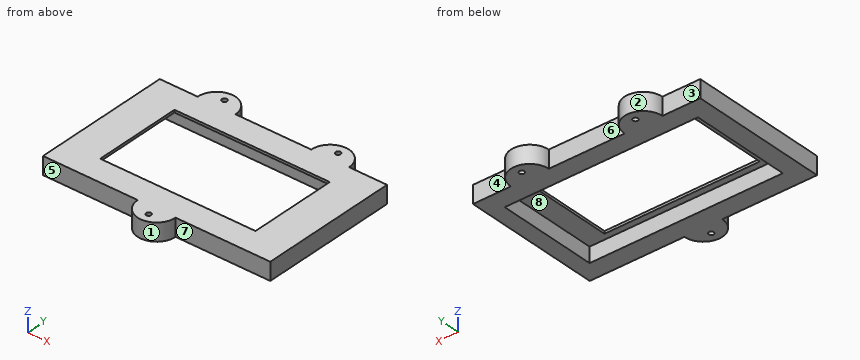
from build123d import *

# Parameters (mm, degrees)
F0_R      = 2
F1_DEPTH  = 25
F3_DEPTH  = 276
F4_R      = 2
F5_DEPTH  = 84.8
F6_R      = 2.5
F7_DEPTH  = 5
F9_DEPTH  = 14
F11_W     = 123
F11_H     = 70
F12_DEPTH = 25
F13_W     = 153
F13_H     = 80
F14_DEPTH = 12
F15_R     = 2
F16_DEPTH = 25


with BuildPart() as f1:
    # F0 (on Top) → F1 (new body)
    with BuildSketch(Plane.XY):
        with BuildLine():
            Line((-51.434658, 66.572686), (-81.434658, 66.572686))
            Line((-81.434658, 66.572686), (-81.434658, -43.427314))
            Line((-81.434658, -43.427314), (-6.434658, -43.427314))
            ThreePointArc((-6.434658, -43.427314), (8.565342, -58.427314), (23.565342, -43.427314))
            Line((23.565342, -43.427314), (98.565342, -43.427314))
            Line((98.565342, -43.427314), (98.565342, 66.572686))
            Line((98.565342, 66.572686), (68.565342, 66.572686))
            ThreePointArc((68.565342, 66.572686), (53.565342, 81.572686), (38.565342, 66.572686))
            Line((38.565342, 66.572686), (-21.434658, 66.572686))
            ThreePointArc((-21.434658, 66.572686), (-36.434658, 81.572686), (-51.434658, 66.572686))
        make_face()
        with Locations((8.565342, -50.927314)):
            Circle(F0_R, mode=Mode.SUBTRACT)
        with Locations((-36.434658, 74.072686)):
            Circle(F0_R, mode=Mode.SUBTRACT)
        with Locations((53.565342, 74.072686)):
            Circle(F0_R, mode=Mode.SUBTRACT)
    extrude(amount=F1_DEPTH)

    # F2 (on face) → F3 (cut)
    with BuildSketch(Plane.YZ.offset(98.565342)):
        with BuildLine():
            Line((43.145373, 0), (22.822686, 0))
            ThreePointArc((22.822686, 0), (11.572686, 11.25), (0.322686, 0))
            Line((0.322686, 0), (-20, 0))
            ThreePointArc((-20, 0), (-41.231841, 11.150842), (-64.902842, 15))
            Line((-64.902842, 15), (-64.902842, -16.413443))
            Line((-64.902842, -16.413443), (88.048215, -16.413443))
            Line((88.048215, -16.413443), (88.048215, 15))
            ThreePointArc((88.048215, 15), (64.377213, 11.150842), (43.145373, 0))
        make_face()
    extrude(amount=-F3_DEPTH, mode=Mode.SUBTRACT)

    # F4 (on face) → F5 (cut)
    with BuildSketch(Plane.XY.offset(25)):
        with Locations((-56.434658, 32.872686)):
            Circle(F4_R)
        with Locations((73.565342, 32.872686)):
            Circle(F4_R)
        with Locations((-56.434658, -9.727314)):
            Circle(F4_R)
        with Locations((73.565342, -9.727314)):
            Circle(F4_R)
    extrude(amount=-F5_DEPTH, mode=Mode.SUBTRACT)

    # F6 (on face) → F7 (cut)
    with BuildSketch(Plane.XY.offset(25)):
        with Locations((-56.434658, 32.872686)):
            Circle(F6_R)
        with Locations((73.565342, 32.872686)):
            Circle(F6_R)
        with Locations((73.565342, -9.727314)):
            Circle(F6_R)
        with Locations((-56.434658, -9.727314)):
            Circle(F6_R)
    extrude(amount=-F7_DEPTH, mode=Mode.SUBTRACT)


with BuildPart() as f9:
    # F8 (on face) → F9 (new body)
    with BuildSketch(Plane.XY.offset(25)):
        with BuildLine():
            Line((-81.434658, -43.427314), (-6.434658, -43.427314))
            ThreePointArc((-6.434658, -43.427314), (8.565342, -58.427314), (23.565342, -43.427314))
            Line((23.565342, -43.427314), (98.565342, -43.427314))
            Line((98.565342, -43.427314), (98.565342, 66.572686))
            Line((98.565342, 66.572686), (68.565342, 66.572686))
            ThreePointArc((68.565342, 66.572686), (53.565342, 81.572686), (38.565342, 66.572686))
            Line((38.565342, 66.572686), (-21.434658, 66.572686))
            ThreePointArc((-21.434658, 66.572686), (-36.434658, 81.572686), (-51.434658, 66.572686))
            Line((-51.434658, 66.572686), (-81.434658, 66.572686))
            Line((-81.434658, 66.572686), (-81.434658, -43.427314))
        make_face()
    extrude(amount=F9_DEPTH)

    # F11 (on face) → F12 (cut)
    with BuildSketch(Plane.XY.offset(39)):
        with Locations((8.565342, 11.572686)):
            Rectangle(F11_W, F11_H)
    extrude(amount=-F12_DEPTH, mode=Mode.SUBTRACT)

    # F13 (on face) → F14 (cut)
    with BuildSketch(Plane(origin=(0, 0, 25), x_dir=(1, 0, 0), z_dir=(0, 0, -1))):
        with Locations((9.565342, -11.572686)):
            Rectangle(F13_W, F13_H)
    extrude(amount=-F14_DEPTH, mode=Mode.SUBTRACT)

    # F15 (on face) → F16 (cut)
    with BuildSketch(Plane.XY.offset(39)):
        with Locations((53.565342, 74.072686)):
            Circle(F15_R)
        with Locations((-36.434658, 74.072686)):
            Circle(F15_R)
        with Locations((8.565342, -50.927314)):
            Circle(F15_R)
    extrude(amount=-F16_DEPTH, mode=Mode.SUBTRACT)


solid = f9.part
The model under review builds one solid part; all positions refer to its coordinate system, in mm. Face numbers are marked on the shaded views. A direction names the side the tool comes from. Give positions to 0.01 mm unless a question says otherwise; leave off trailing zeros. Order: outer loops, then holes, each group sorted by start corner. A loop starts at its lowest first (then second) coordinate and runs counter-clockwise, first axis right, second up. Notation, with made-up numbers: M -11.75,63.25 L 6.25,63.25 A6 cw 6.25,68.25 Z; hole C 35,50.25 d9. An arc over 180 degrees is marked long. Answer in a Markdown table with one row per item. Add a question column.
1. Add section A-A on y = 22. State the section outline as (x, z) points, plus the area to 3 significant figures.
2. Add section D-D on x = -60. State the section outline as (y, z) points, plus the area to 3 significant figures.
3. To check wall thickness, follow line 1 along X through (y, z) = (9, 30.5); line 2 along Y through (x, z) = (-8, 30.25); line 3 along Y through (x, z) = (52, 30.25). State the ranges of each line that lie inside material, in increasing order.
4. Mouldability with a two-part tool opening along X and no side actions: class the marked faces 1, 2 and 3 as released by +X, released by -X, zero draft, split by the parting line, or undercut.
5. Machinability: for the marked faces 4, 5, 6, 7 and 8, which of the approach directions +Z, -Z, +X, -X, +Y, -Y give a long, thin tool a straight path to every point of the face, cutting with its end or side? Answer none if there is none.
6. Add section C-C on z = 32. State the section outline as (x, y) points.
7. Add section B-B on x = 63. State the section outline as (y, z) points, plus the area to 3 significant figures.
8. For pin 1 Ø7 at (x, z) = (-35.5, 29) entering from -Y; pin 2 Ø0.6 at (x, z) = (-6.5, 38) entering from +Y; pin 3 Ø1 at (x, z) = (17, 36) entering from -Y; pin 4 Ø2.5 at (x, y) = (8.57, -50.93) entering from -Z, all flat-tipped, find the tip position at first contact; note any pin that passes through.
The answers:
| question | item | result |
|---|---|---|
| 1 | outline | M -81.43,25 L -66.93,25 L -66.93,37 L -52.93,37 L -52.93,39 L -81.43,39 Z; M 70.07,37 L 86.07,37 L 86.07,25 L 98.57,25 L 98.57,39 L 70.07,39 Z |
| 1 | area | 438 mm2 |
| 2 | outline | M -43.43,25 L -28.43,25 L -28.43,37 L 51.57,37 L 51.57,25 L 66.57,25 L 66.57,39 L -43.43,39 Z |
| 2 | area | 580 mm2 |
| 3 | line 1 | -81.43 to -66.93, 86.07 to 98.57 |
| 3 | line 2 | -43.43 to -28.43, 51.57 to 66.57 |
| 3 | line 3 | -43.43 to -28.43, 51.57 to 72.83, 75.32 to 81.49 |
| 4 | face 1 | split by the parting line |
| 4 | face 2 | undercut |
| 4 | face 3 | zero draft |
| 5 | face 4 | +Z, -Z, +X, +Y |
| 5 | face 5 | +Z, -Z, -X, -Y |
| 5 | face 6 | +Z, -Z, +Y |
| 5 | face 7 | +Z, -Z, +X, -Y |
| 5 | face 8 | -Z |
| 6 | outline | M -81.43,-43.43 L -6.43,-43.43 A15 ccw 23.57,-43.43 L 98.57,-43.43 L 98.57,66.57 L 68.57,66.57 A15 ccw 38.57,66.57 L -21.43,66.57 A15 ccw -51.43,66.57 L -81.43,66.57 Z; hole M -66.93,-28.43 L 86.07,-28.43 L 86.07,51.57 L -66.93,51.57 Z; hole C -36.43,74.07 d4; hole C 8.57,-50.93 d4; hole C 53.57,74.07 d4 |
| 7 | outline | M -43.43,25 L -28.43,25 L -28.43,37 L -23.43,37 L -23.43,39 L -43.43,39 Z; M 46.57,37 L 51.57,37 L 51.57,25 L 78.23,25 L 78.23,39 L 46.57,39 Z |
| 7 | area | 603 mm2 |
| 8 | pin 1 | y = -43.43 |
| 8 | pin 2 | y = 66.57 |
| 8 | pin 3 | y = -56.16 |
| 8 | pin 4 | through |
